Input: dimensioned drawing with shaded views. Units: mm. Origin: part minimum x, y, z. A direction names the side the tool comes from. Round coordinates to 2 decimals unless told otherwise and drop trailing zeros. Loops run counter-clockwise (first coordinate to the right, second up) from the corner with the lowest first, then second, coordinate; pieces in that order, holes last. Notation, with made-up numbers: (4.25, -29) -> (26.25, -29) arc R16 cw to (26.25, -19) -> close; hole circle Ø11 at (56.5, 82.5). An arc over 180 degrees is marked (long way). Answer as a JSON object with one key per item and string values.
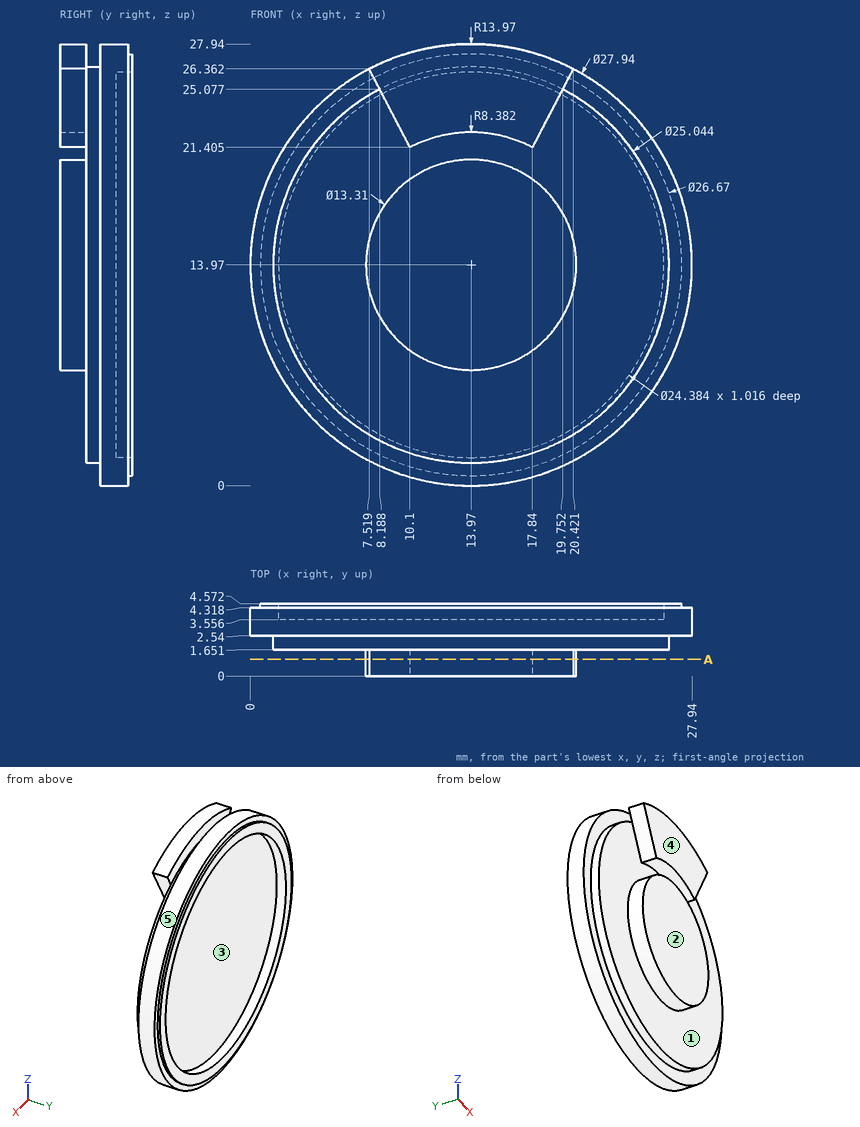
1) Ray query, probe 1 along Y at (x, z) = (10.5, 26.5); probe 2 along Z at (x, y) = (13.75, 4.2). Return the intervals inside material, ascending.
Output:
{"probe 1": "y = 0 to 1.65, 2.54 to 4.57", "probe 2": "z = 0 to 1.78, 26.16 to 27.94"}
2) Contact query for flat-ended pins moving along their axis: P1, Ø2, axis at x = 24, y = 1.5, coming from the +Z side (1 decimal); P2, Ø7.5, axis at x = 15, z = 13.5, coming from the +Y side. Output: stop coordinate, or through.
Output:
{"P1": "stops at z = 22.6", "P2": "stops at y = 3.56"}
3) Section A-A, the plane y = 1.05. Output: boundary loops of the cut face in (x, z) (1 decimal), plus the area to 3 significant figures.
Output:
{"outline": "circle Ø13.3 at (14, 14); (7.5, 26.4) -> (10.1, 21.4) arc R8.4 cw to (17.8, 21.4) -> (20.4, 26.4) arc R14 ccw to start", "area": "199 mm^2"}
4) Draft query along X for the marked faces 3, 4 and 5. Return one class per face: +X half, -X half, draft (parallel to the pull), parting line (faces both ways), or undercut.
Output:
{"face 3": "undercut", "face 4": "draft", "face 5": "parting line"}
5) Reachability of the marked faces 1 and 2 from +Z, -Z, +X, -X, +Y, -Y: full face, straight path, thin tool, end or side. Return the list, or none.
Output:
{"face 1": "-Y", "face 2": "+Z, -Z, +X, -X, -Y"}
